Design review of the part shown in the three views and the two pictorial views. Dimensions are in mm from the part's minimum x, y and z. A direction names the side the tool comes from. Round coordinates to 2 decimals unless told otherwise and drop trailing zeros. Order: outer loops, then holes, each group sorted by start corner. A loop starts at its lowest first (then second) coordinate and runs counter-clockwise, first axis right, second up.
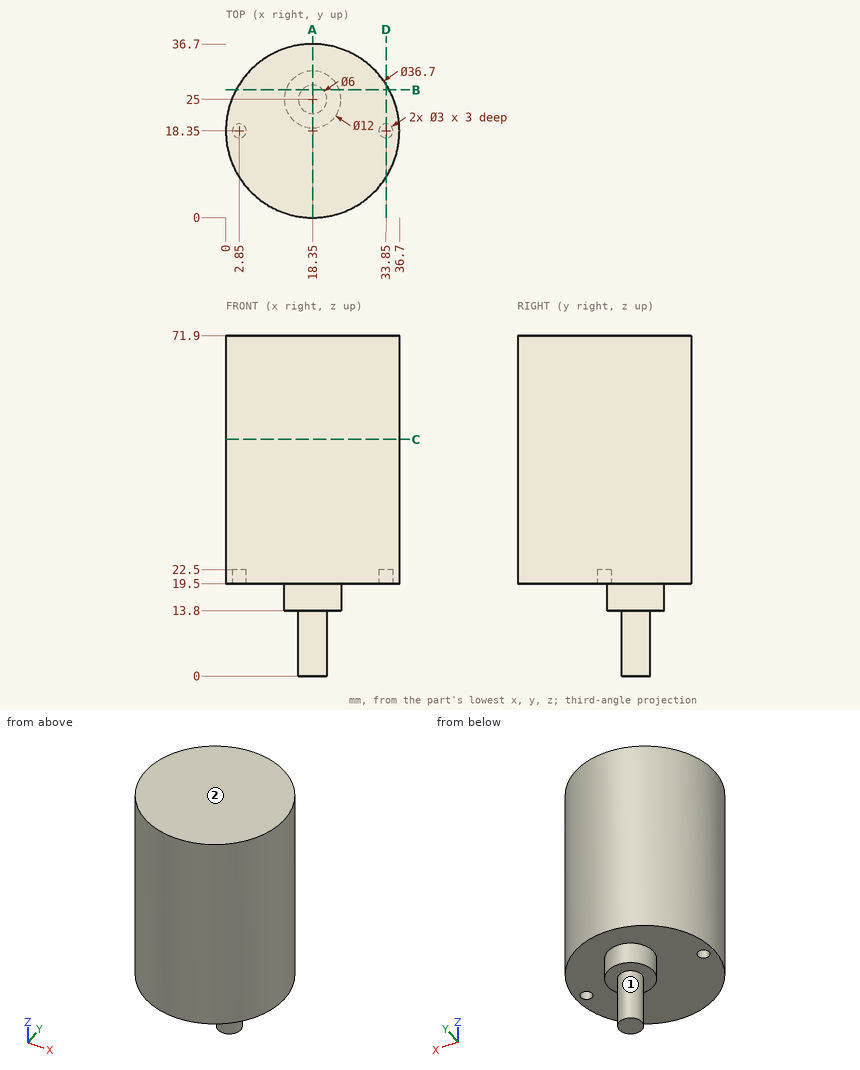
(1) Consider section D-D (x = 33.85). Write out the cut boundary in (y, z), and give its area (3 significant figures).
Data:
outline: (8.53, 19.5) - (16.85, 19.5) - (16.85, 22.5) - (19.85, 22.5) - (19.85, 19.5) - (28.17, 19.5) - (28.17, 71.9) - (8.53, 71.9) - close
area: 1,020 mm2
(2) Consider section A-A (x = 18.35). Write out the cut boundary in (y, z).
Data:
outline: (0, 19.5) - (19, 19.5) - (19, 13.8) - (22, 13.8) - (22, 0) - (28, 0) - (28, 13.8) - (31, 13.8) - (31, 19.5) - (36.7, 19.5) - (36.7, 71.9) - (0, 71.9) - close
(3) To check wall thickness, follow probe 1 along X at (y, z) = (18, 20); probe 2 along Z at (x, y) = (10.5, 23); probe 3 along Y at (x, z) = (33.85, 20.85). State the ranges of each line that lie inside material, in increasing order.
Data:
probe 1: x = 0 to 1.39, 4.31 to 32.39, 35.31 to 36.7
probe 2: z = 19.5 to 71.9
probe 3: y = 8.53 to 16.85, 19.85 to 28.17
(4) Consider section B-B (y = 27). Write out the cut boundary in (x, z).
Data:
outline: (2.17, 19.5) - (12.69, 19.5) - (12.69, 13.8) - (16.11, 13.8) - (16.11, 0) - (20.59, 0) - (20.59, 13.8) - (24.01, 13.8) - (24.01, 19.5) - (34.53, 19.5) - (34.53, 71.9) - (2.17, 71.9) - close
(5) For the marked faces 1 and 2, list the 3-axis set-ups (+Z, -Z, +X, -X, +Y, -Y) from which the entire face can be reached by the end or side of a thin tool; tool diameter is ignored.
Data:
face 1: -Z
face 2: +Z, +X, -X, +Y, -Y
(6) Insertion check: pin 1 (1.5 mm diameter, centred on x = 8.5, y = 8, fed in from -Z); pin 2 (1 mm diameter, centred on y = 27, z = 28.5, fed in from +X); pin 3 (11 mm diameter, centred on x = 13, y = 18, fed in from -Z). Each pin has a flat end and moves straight along its axis. Give the tip position at first contact, or say it passes through.
Data:
pin 1: stops at z = 19.5
pin 2: stops at x = 34.79
pin 3: stops at z = 13.8
(7) Consider section C-C (z = 50). Write out the cut boundary in (x, y).
Data:
outline: circle Ø36.7 at (18.35, 18.35)
